Geometry: final body of the model. Coordinates: model frame, mm. A direction names the side the tool comes from. Round coordinates to 2 decimals unless told otherwise and drop trailing zeros. Loops run counter-clockwise (first coordinate to the right, second up) from the corner with the lowest first, then second, coordinate; pieces in that order, holes last. Notation, with made-up numbers: M -21,18 L -8,18 A14 cw -8,23 Z; hole C -14,55.25 d9. An arc over 180 degrees is marked long. Answer as a JSON object with one key per item and string values.
```python
from build123d import *

# Parameters (mm, degrees)
F0_R     = 28.575
F1_DEPTH = 20.1168


with BuildPart() as f1:
    # F0 (on Front) → F1 (new body, symmetric)
    with BuildSketch(Plane.XZ):
        Circle(F0_R)
        with BuildLine():
            ThreePointArc((-14.2875, 0), (-2.449257, 14.076001), (13.447765, 4.826))
            Line((13.447765, 4.826), (18.5293, 4.826))
            Line((18.5293, 4.826), (18.5293, 0))
            Line((18.5293, 0), (18.5293, -4.826))
            Line((18.5293, -4.826), (13.447765, -4.826))
            ThreePointArc((13.447765, -4.826), (-2.449257, -14.076001), (-14.2875, 0))
        make_face(mode=Mode.SUBTRACT)
    extrude(amount=F1_DEPTH, both=True)


solid = f1.part
```
1) Cut plane A-A on x = 0. Return the cut outline in (y, z) (1 decimal).
Geometry results:
{"outline": "M -20.1,-28.6 L 20.1,-28.6 L 20.1,-14.3 L -20.1,-14.3 Z; M -20.1,14.3 L 20.1,14.3 L 20.1,28.6 L -20.1,28.6 Z"}
2) Pull-direction query (X, two-part tool) for faces 1 (the face through (16, 0, -4.826)), 2 (the face through (-13, -20.117, 7)), 3 (the face through (-28.547, -0.282, 1.256)), 4 (the face through (16, 0, 4.826)); classes: +X half, -X half, draft (parallel to the pull), parting line (faces both ways), or undercut.
Geometry results:
{"face 1": "undercut", "face 2": "draft", "face 3": "parting line", "face 4": "undercut"}
3) Line query: probe 1 along Z at (x, y) = (0, 14.5) (1 decimal); probe 2 along Z at (x, y) = (-1.5, 11.5); probe 3 along X at (y, z) = (-10, -6). Output: solid intervals per line, ascending.
Geometry results:
{"probe 1": "-28.6 to -14.3, 14.3 to 28.6", "probe 2": "-28.54 to -14.21, 14.21 to 28.54", "probe 3": "-27.94 to -12.97, 12.97 to 27.94"}
4) First-contact query: pin 1 (6 mm diameter, centred on y = 4.5, z = 16.5, fed in from -X); pin 2 (5 mm diameter, centred on y = 2.5, z = 17, fed in from +X); pin 3 (5.5 mm diameter, centred on x = 17, y = 7, fed in from -Z). Flat tips, straight axial feed; report the tip coordinate or a pass-through.
Geometry results:
{"pin 1": "x = -25.18", "pin 2": "x = 24.62", "pin 3": "z = -24.77"}
5) Cut plane D-D on z = -15.5. Return the cut outline in (x, y).
Geometry results:
{"outline": "M -24.01,-20.12 L 24.01,-20.12 L 24.01,20.12 L -24.01,20.12 Z"}
6) Set-up query: faces 5 (the face through (-13, 20.117, 7)), 6 (the face through (18.529, 0, 0)). Return all of +Z, -Z, +X, -X, +Y, -Y with unobstructed straight access to the full face (end or side cutting, diameter ignored); none if empty.
Geometry results:
{"face 5": "+Z, -Z, +X, -X, +Y", "face 6": "+Y, -Y"}
7) Cut plane B-B on z = 7. Return the cut outline in (x, y).
Geometry results:
{"outline": "M -27.7,-20.12 L -12.46,-20.12 L -12.46,20.12 L -27.7,20.12 Z; M 12.46,-20.12 L 27.7,-20.12 L 27.7,20.12 L 12.46,20.12 Z"}
